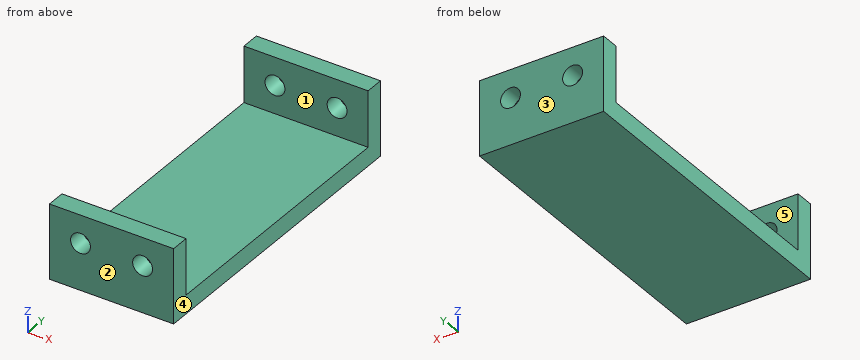
```python
from build123d import *

# Parameters (mm, degrees)
SKETCH_1_W          = 20
SKETCH_1_H          = 50
EXTRUDE_1_DEPTH     = 12
SKETCH_2_W          = 20
SKETCH_2_H          = 44
CUT_EXTRUDE_1_DEPTH = 9
SKETCH_3_R          = 1.6
CUT_EXTRUDE_2_DEPTH = 51


with BuildPart() as part:
    # 草图1 → 凸台-拉伸1 (new body)
    with BuildSketch(Plane.XY):
        with Locations((-5.803858521, -0.908360129)):
            Rectangle(SKETCH_1_W, SKETCH_1_H)
    extrude(amount=EXTRUDE_1_DEPTH)

    # 草图2 → 切除-拉伸1 (cut)
    with BuildSketch(Plane.XY.offset(12)):
        with Locations((-5.803858521, -0.908360129)):
            Rectangle(SKETCH_2_W, SKETCH_2_H)
    extrude(amount=-CUT_EXTRUDE_1_DEPTH, mode=Mode.SUBTRACT)

    # 草图3 → 切除-拉伸2 (cut, through all)
    with BuildSketch(Plane(origin=(0, 24.091639871, 0), x_dir=(1, 0, 0), z_dir=(0, 1, 0))):
        with Locations((-10.803858521, -7.5)):
            Circle(SKETCH_3_R)
        with Locations((-0.803858521, -7.5)):
            Circle(SKETCH_3_R)
    extrude(amount=-CUT_EXTRUDE_2_DEPTH, mode=Mode.SUBTRACT)


solid = part.part
```
The model under review builds one solid part; all positions refer to its coordinate system, in mm. Face numbers are marked on the shaded views. A direction names the side the tool comes from. Round coordinates to 2 decimals unless told otherwise and drop trailing zeros. Write each loop counter-clockwise with the first axis right and the second up, starting at its lowest first coordinate (ties: lowest second). Pieces come first, ordered by that corner, then holes.
(1) Wall thickness on L1, parallel to X at y = -23.9, z = 7.5; L2, parallel to Y at x = -4, z = 8.75; L3, parallel to X at y = 21.5, z = 7: over which ranges is each line inside the solid? List them lowest first.
(2) Mouldability with a two-part tool opening along Y and no side actions: class the marked faces 3, 4 and 5 as +Y half, -Y half, draft (parallel to the pull), parting line (faces both ways), or undercut.
(3) We need section A-A on z = 10.25. Give the boundary of the cut face in (x, y), and give its area (3 significant figures).
(4) We need section D-D on x = -13.5. Give the boundary of the cut face in (y, z).
(5) We need section C-C on z = 7.5. Give the boundary of the cut face in (x, y).
(6) Insertion check: pin 1 (2.5 mm diameter, centred on x = -10.8, z = 7.5, fed in from +Y); pin 2 (1 mm diameter, centred on x = -6.5, y = 0.5, fed in from +Z). Each pin has a flat end and moves straight along its axis. Give the tip position at first contact, or say it passes through.
(7) We need section B-B on x = -1.75. Give the boundary of the cut face in (y, z).
(8) Machinability: for the marked faces 1 and 2, which of the approach directions +Z, -Z, +X, -X, +Y, -Y give a long, thin tool a straight path to every point of the face, cutting with its end or side? Answer none if there is none.
Findings below:
1. L1: x = -15.8 to -12.4, -9.2 to -2.4, 0.8 to 4.2
1. L2: y = -25.91 to -22.91, 21.09 to 24.09
1. L3: x = -15.8 to -12.32, -9.28 to -2.32, 0.72 to 4.2
2. face 3: +Y half
2. face 4: draft
2. face 5: undercut
3. outline: (-15.8, -25.91) - (4.2, -25.91) - (4.2, -22.91) - (-15.8, -22.91) - close; (-15.8, 21.09) - (4.2, 21.09) - (4.2, 24.09) - (-15.8, 24.09) - close
3. area: 120 mm2
4. outline: (-25.91, 0) - (24.09, 0) - (24.09, 12) - (21.09, 12) - (21.09, 3) - (-22.91, 3) - (-22.91, 12) - (-25.91, 12) - close
5. outline: (-15.8, -25.91) - (-12.4, -25.91) - (-12.4, -22.91) - (-15.8, -22.91) - close; (-15.8, 21.09) - (-12.4, 21.09) - (-12.4, 24.09) - (-15.8, 24.09) - close; (-9.2, -25.91) - (-2.4, -25.91) - (-2.4, -22.91) - (-9.2, -22.91) - close; (-9.2, 21.09) - (-2.4, 21.09) - (-2.4, 24.09) - (-9.2, 24.09) - close; (0.8, -25.91) - (4.2, -25.91) - (4.2, -22.91) - (0.8, -22.91) - close; (0.8, 21.09) - (4.2, 21.09) - (4.2, 24.09) - (0.8, 24.09) - close
6. pin 1: passes through
6. pin 2: stops at z = 3
7. outline: (-25.91, 0) - (24.09, 0) - (24.09, 6.21) - (21.09, 6.21) - (21.09, 3) - (-22.91, 3) - (-22.91, 6.21) - (-25.91, 6.21) - close; (-25.91, 8.79) - (-22.91, 8.79) - (-22.91, 12) - (-25.91, 12) - close; (21.09, 8.79) - (24.09, 8.79) - (24.09, 12) - (21.09, 12) - close
8. face 1: +Z, +X, -X
8. face 2: +Z, -Z, +X, -X, -Y
